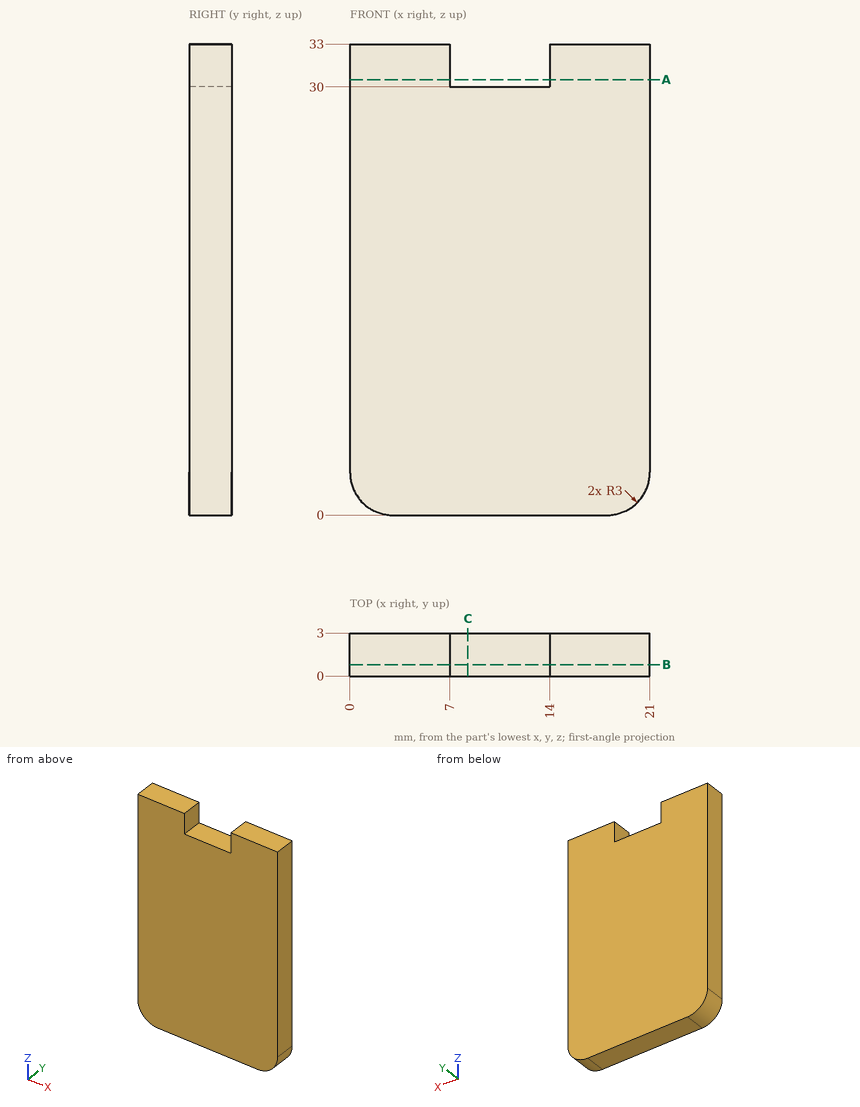
Source: three-view drawing plus pictorial views. Frame: mm from the lowest corner of the part. Coordinates: 2 decimals unless noted, no trailing zeros. Order: outer loops, then holes, each group sorted by start corner. A loop starts at its lowest first (then second) coordinate and runs counter-clockwise, first axis right, second up.
Item 1: Cut plane A-A (z = 30.5). Return loops of the section in (x, y), plus the area to 3 significant figures.
Output values:
outline: (0, 0) - (7, 0) - (7, 3) - (0, 3) - close; (14, 0) - (21, 0) - (21, 3) - (14, 3) - close
area: 42.0 mm2
Item 2: First-contact query: P1, Ø0.9, axis at x = 11.5, y = 1.5, coming from the +Z side. Flat tip, straight axial feed; report the tip coordinate or a pass-through.
Output values:
P1: stops at z = 30
Item 3: Material intervals for line 1 (Z direction, x = 13.25, y = 2.15); line 2 (Z direction, x = 19.25, y = 0.2); line 3 (X direction, y = 1.3, z = 2.5), sorted ascending.
Output values:
line 1: z = 0 to 30
line 2: z = 0.27 to 33
line 3: x = 0.04 to 20.96
Item 4: Cut plane B-B (y = 0.8). Return loops of the section in (x, z), plus the area to 3 significant figures.
Output values:
outline: (0, 3) arc R3 ccw to (3, 0) - (18, 0) arc R3 ccw to (21, 3) - (21, 33) - (14, 33) - (14, 30) - (7, 30) - (7, 33) - (0, 33) - close
area: 668 mm2
Item 5: Cut plane C-C (x = 8.25). Return loops of the section in (y, z).
Output values:
outline: (0, 0) - (3, 0) - (3, 30) - (0, 30) - close
